from build123d import *

# Parameters (mm, degrees)
F1_DEPTH       = 12.7
F3_DEPTH       = 254
F5_DEPTH       = 254
F5_DEPTH_BACK  = 25.4
F6_R           = 19.9026330237
F7_DEPTH       = 0.254
F7_DEPTH_BACK  = 15.24
F8_R           = 6.35
F9_DEPTH       = 25.4
F10_DEPTH      = 12.7
F10_DEPTH_BACK = 76.2
F11_R          = 28.575
F12_DEPTH      = 2.54
F12_DEPTH_BACK = 25.4
F13_R          = 41.275
F14_DEPTH      = 101.6
F14_DEPTH_BACK = 25.4


with BuildPart() as f1:
    # F0 (on Right) → F1 (new body, symmetric)
    with BuildSketch(Plane.YZ):
        with BuildLine():
            Line((-25.4, 50.8), (-15.24, 11.43))
            ThreePointArc((-15.24, 11.43), (-19.05, 0), (-15.24, -11.43))
            Line((-15.24, -11.43), (-25.4, -50.8))
            Line((-25.4, -50.8), (-11.8797372622, -127))
            Line((-11.8797372622, -127), (0, -127))
            Line((0, -127), (11.8797372622, -127))
            Line((11.8797372622, -127), (25.4, -50.8))
            Line((25.4, -50.8), (15.24, -11.43))
            ThreePointArc((15.24, -11.43), (19.05, 0), (15.24, 11.43))
            Line((15.24, 11.43), (25.4, 50.8))
            Line((25.4, 50.8), (11.8797372622, 127))
            Line((11.8797372622, 127), (0, 127))
            Line((0, 127), (-11.8797372622, 127))
            Line((-11.8797372622, 127), (-25.4, 50.8))
        make_face()
    extrude(amount=F1_DEPTH, both=True)

    # F2 (on Top) → F3 (cut)
    with BuildSketch(Plane.XY):
        Polygon((15.0384465232, 34.2237874866), (-14.059139771, 34.2237874866), (15.0384465232, -126.2663410758), align=None)
    extrude(amount=-F3_DEPTH, mode=Mode.SUBTRACT)

    # F4 (on Top) → F5 (cut, two sides)
    with BuildSketch(Plane.XY) as f5_sk:
        Polygon((7.2715352289, 50.541035831), (-13.9147825539, -30.9769567102), (33.8218561163, -30.9769567102), align=None)
    extrude(amount=F5_DEPTH, mode=Mode.SUBTRACT)
    extrude(f5_sk.sketch, amount=-F5_DEPTH_BACK, mode=Mode.SUBTRACT)

    # F6 (on Right) → F7 (join, two sides)
    with BuildSketch(Plane.YZ) as f7_sk:
        Circle(F6_R)
    extrude(amount=F7_DEPTH)
    extrude(f7_sk.sketch, amount=-F7_DEPTH_BACK)

    # F8 (on face) → F9 (cut)
    with BuildSketch(Plane.YZ.offset(0.254)):
        Circle(F8_R)
    extrude(amount=-F9_DEPTH, mode=Mode.SUBTRACT)

    # F8 (on face) → F10 (join, two sides)
    with BuildSketch(Plane.YZ.offset(0.254)) as f10_sk:
        Circle(F8_R)
    extrude(amount=F10_DEPTH)
    extrude(f10_sk.sketch, amount=-F10_DEPTH_BACK)

    # F11 (on face) → F12 (join, two sides)
    with BuildSketch(Plane(origin=(-75.946, 0, 0), x_dir=(0, -1, 0), z_dir=(-1, 0, 0))) as f12_sk:
        Circle(F11_R)
    extrude(amount=F12_DEPTH)
    extrude(f12_sk.sketch, amount=-F12_DEPTH_BACK)

    # F13 (on face) → F14 (join, two sides)
    with BuildSketch(Plane(origin=(-78.486, 0, 0), x_dir=(0, -1, 0), z_dir=(-1, 0, 0))) as f14_sk:
        Circle(F13_R)
    extrude(amount=F14_DEPTH)
    extrude(f14_sk.sketch, amount=-F14_DEPTH_BACK)

    # F15 (on Front) → F16 (revolve)
    with BuildSketch(Plane.XZ):
        with BuildLine():
            Line((34.7278043628, 0), (0, 0))
            Line((0, 0), (0, -12.609985657))
            add(Edge.make_bspline(
                [(34.7278043628, 0), (32.128238571, -3.207452008), (25.8473025253, -10.9571312029), (9.5513516448, -11.9992064822), (0, -12.609985657)],
                knots=[0, 0, 0, 0, 0.4138819075, 1, 1, 1, 1], degree=3))
        make_face()
    revolve(axis=Axis((17.3639021814, 0, 0), (1, 0, 0)))


solid = f1.part
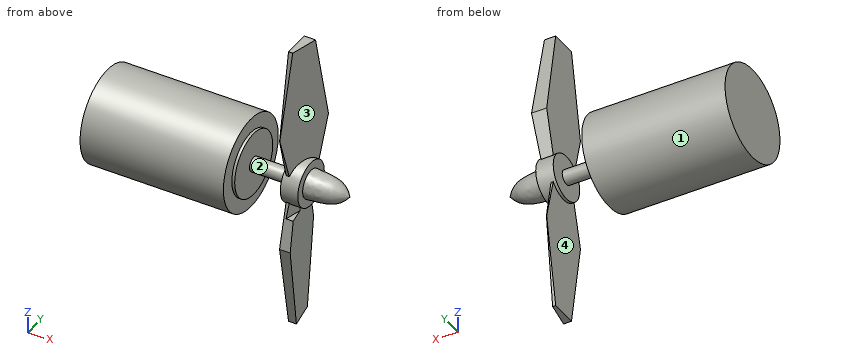
CAD build for the part. Positions are in the model's coordinates, mm. Face numbers are marked on the shaded views. Round coordinates to 2 decimals unless told otherwise and drop trailing zeros. Order: outer loops, then holes, each group sorted by start corner. A loop starts at its lowest first (then second) coordinate and runs counter-clockwise, first axis right, second up. Notation, with made-up numbers: (78, 20) -> (128, 20) arc R19 ccw to (128, 38) -> close; hole circle Ø5 at (-23.5, -30). An arc over 180 degrees is marked (long way). Write item = value, one per line. Start each with the question number.
(1) Pin check, flat tips, straight feed: P1, Ø1.5, axis at x = -98, y = 2.5, coming from the -Z side; P2, Ø5, axis at y = 16, z = -48, coming from the +X side; P3, Ø12, axis at y = 22.5, z = 7, coming from the +X side. Stop position of each tip, or through.
(2) Cut at B-B, the plane z = 97. List the corners of the cut face in (x, y).
(3) Cut at D-D, the plane z = -70. List the corners of the cut face in (x, y).
(4) Pull direction X, two halves, no side cores. Call the marked faces 1, 2, 3 and 4: released by +X, released by -X, zero draft, split by the parting line, or undercut.
(5) Cut at A-A, the plane x = -87. List the corners of the cut face in (y, z) (3 decimals), then the cut area to 3 significant figures.
(6) Cut at C-C, the plane x = -27. List the corners of the cut face in (y, z), then the cut area to 3 significant figures.
(7) Probe line 1 (X direction, y = -20, z = 23); line 2 (X direction, y = 12, z = 95); line 3 (X direction, y = -10, z = -40). List the from-to ranges inside material, lowest first. Write a range as [from, to].
Model answer:
q1.P1 = -41.24
q1.P2 = -10.3
q1.P3 = 0.25
q2.outline = (-12.7, -17.2) -> (-10.33, -17.2) -> (-1.39, 17.2) -> (-12.7, 17.2) -> close
q3.outline = (-12.7, -21.99) -> (-3.87, -21.99) -> (-11.84, 21.99) -> (-12.7, 21.99) -> close
q4.face_1 = zero draft
q4.face_2 = undercut
q4.face_3 = released by +X
q4.face_4 = undercut
q5.outline = circle Ø82.55 at (0, 0)
q5.area = 5,350 mm2
q6.outline = circle Ø12.7 at (0, 0)
q6.area = 127 mm2
q7.line_1 = [-180.09, -53.09]
q7.line_2 = [-12.7, -2.75]
q7.line_3 = [-180.09, -53.09], [-12.7, -6.04]
